Design review of the part built by this model. Coordinates are the model's own, in mm. Coordinates: 2 decimals unless noted, no trailing zeros. Order: outer loops, then holes, each group sorted by start corner. A loop starts at its lowest first (then second) coordinate and runs counter-clockwise, first axis right, second up. Notation, with made-up numbers: M 50,86.25 L 67,86.25 A24 ccw 67,118.25 Z; hole C -28.5,-19.5 d1. An arc over 180 degrees is marked long. Answer as a JSON object with one key per item and string values.
from build123d import *

# Parameters (mm, degrees)
F0_W     = 63.5
F0_H     = 139.7
F1_DEPTH = 12.7
F3_DEPTH = 25.4
F4_R     = 3.175
F5_DEPTH = 25.4


with BuildPart() as f1:
    # F0 (on Front) → F1 (new body)
    with BuildSketch(Plane.XZ):
        with Locations((-20.063438, 21.341896)):
            Rectangle(F0_W, F0_H)
    extrude(amount=F1_DEPTH)

    # F2 (on face) → F3 (cut)
    with BuildSketch(Plane.XZ.offset(12.7)):
        Polygon((-51.813438, 40.391896), (-20.063438, 91.191896), (-51.813438, 91.191896), align=None)
        Polygon((11.686562, 91.191896), (-20.063438, 91.191896), (11.686562, 40.391896), align=None)
    extrude(amount=-F3_DEPTH, mode=Mode.SUBTRACT)

    # F4 (on face) → F5 (cut)
    with BuildSketch(Plane(origin=(0, 0, -48.508104), x_dir=(1, 0, 0), z_dir=(0, 0, -1))):
        with Locations((-19.809052, 6.35)):
            Circle(F4_R)
    extrude(amount=-F5_DEPTH, mode=Mode.SUBTRACT)


solid = f1.part
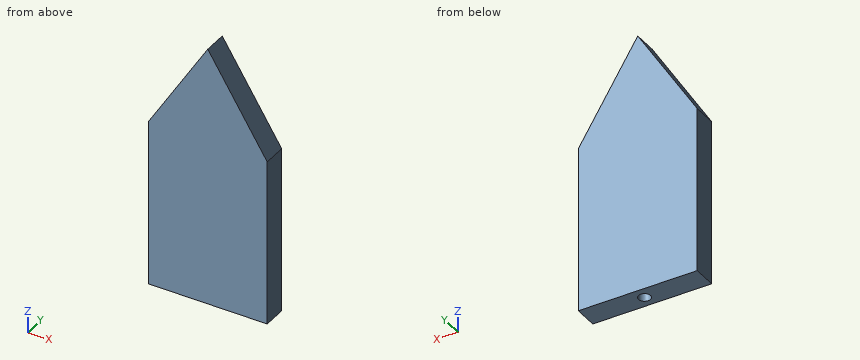
1) Add section C-C (x = -35.5). State the section outline as (y, z) points.
Taken from the geometry:
{"outline": "M -12.7,-48.51 L 0,-48.51 L 0,66.49 L -12.7,66.49 Z"}
2) Insertion check: pin 1 Ø5 at (x, y) = (-19, -6) entering from -Z; pin 2 Ø5 at (y, z) = (-2.5, 56.5) entering from +X. Each pin has a flat end and moves straight along its axis. Give the tip position at first contact, or say it passes through.
Taken from the geometry:
{"pin 1": "stops at z = -48.51", "pin 2": "stops at x = 3.18"}
3) Add section B-B (x = -5.5). State the section outline as (y, z) points, and give its area (3 significant figures).
Taken from the geometry:
{"outline": "M -12.7,-48.51 L 0,-48.51 L 0,67.89 L -12.7,67.89 Z", "area": "1,480 mm2"}
4) Add section A-A (y = -6.35). State the section outline as (x, z) points, and give its area (3 significant figures).
Taken from the geometry:
{"outline": "M -51.81,-48.51 L -22.98,-48.51 L -22.98,-23.11 L -16.63,-23.11 L -16.63,-48.51 L 11.69,-48.51 L 11.69,40.39 L -20.06,91.19 L -51.81,40.39 Z", "area": "7,100 mm2"}
5) To check wall thickness, follow L1, parallel to X at y = -6.35, z = -34; L2, parallel to Z at x = -29, y = -3.75; L3, parallel to Z at x = 7.5, y = -11. State the ranges of each line that lie inside material, in increasing order.
Taken from the geometry:
{"L1": "x = -51.81 to -22.98, -16.63 to 11.69", "L2": "z = -48.51 to 76.89", "L3": "z = -48.51 to 47.09"}
